```python
from build123d import *

# Parameters (mm, degrees)
ESQUISSE1_R             = 9
BOSS_EXTRU_1_DEPTH      = 23
ESQUISSE2_R             = 9
ESQUISSE2_R_2           = 4.5
ENL_V_MAT_EXTRU_2_DEPTH = 27.286878856
ESQUISSE3_R             = 1.5
ENL_V_MAT_EXTRU_3_DEPTH = 5
ESQUISSE4_R             = 2
ENL_V_MAT_EXTRU_4_DEPTH = 5


with BuildPart() as part:
    # Esquisse1 → Boss.-Extru.1 (new body)
    with BuildSketch(Plane(origin=(0, 0, 0), x_dir=(1, 0, 0), z_dir=(0, 1, 0))):
        with Locations(Location((0, 0, 0), (0, 0, 270))):
            Circle(ESQUISSE1_R)
    extrude(amount=BOSS_EXTRU_1_DEPTH)

    # Esquisse2 → Enlèv. mat.-Extru.2 (cut, through all)
    with BuildSketch(Plane(origin=(0, 0, 0), x_dir=(-1, 0, 0), z_dir=(0, -1, 0))):
        Circle(ESQUISSE2_R)
        with Locations(Location((0, 0, 0), (0, 0, 90))):
            Circle(ESQUISSE2_R_2, mode=Mode.SUBTRACT)
    extrude(amount=-ENL_V_MAT_EXTRU_2_DEPTH, mode=Mode.SUBTRACT)

    # Esquisse3 → Enlèv. mat.-Extru.3 (cut)
    with BuildSketch(Plane(origin=(0, 0, 0), x_dir=(-1, 0, 0), z_dir=(0, -1, 0))):
        with Locations(Location((0, 0, 0), (0, 0, 90))):
            Circle(ESQUISSE3_R)
    extrude(amount=-ENL_V_MAT_EXTRU_3_DEPTH, mode=Mode.SUBTRACT)

    # Esquisse4 → Enlèv. mat.-Extru.4 (cut)
    with BuildSketch(Plane(origin=(0, 23, 0), x_dir=(1, 0, 0), z_dir=(0, 1, 0))):
        with Locations(Location((0, 0, 0), (0, 0, 270))):
            Circle(ESQUISSE4_R)
    extrude(amount=-ENL_V_MAT_EXTRU_4_DEPTH, mode=Mode.SUBTRACT)


solid = part.part
```
The model under review builds one solid part; all positions refer to its coordinate system, in mm. A direction names the side the tool comes from. Round coordinates to 2 decimals unless told otherwise and drop trailing zeros. Write each loop counter-clockwise with the first axis right and the second up, starting at its lowest first coordinate (ties: lowest second). Pieces come first, ordered by that corner, then holes. Notation, with made-up numbers: M 37.25,51 L 52.25,51 A19 cw 52.25,56 Z; hole C 86.25,41 d8. An arc over 180 degrees is marked long. Use CSV: the item, a comma, the result in double quotes. Start each with the question number.
(1) We need section A-A, the plane z = 0. State the section outline as (x, y) points, then the cut area to 3 significant figures.
(2) We need section D-D, the plane y = 15. State the section outline as (x, z) points, then the cut area to 3 significant figures.
(3) For line 1 along X through (y, z) = (1.95, 0); line 2 along X through (y, z) = (20.05, 0); line 3 along Y through (x, z) = (-1.5, 1), list the stretches that pass through material, from the lowest coordinate up.
(4) Tool access review of faces 1 (the face through (-2, 23, 1)), 2 (the face through (0, 5, 0)): name each direction out of +Z, -Z, +X, -X, +Y, -Y from which nothing blocks a thin tool from reaching the whole face with its end or side.
(5) We need section C-C, the plane y = 20.5. State the section outline as (x, z) points, then the cut area to 3 significant figures.
(6) We need section B-B, the plane x = 0. State the section outline as (y, z) points.
(7) Clearance check with flat-ended pins moving along their axes: P1, Ø4, axis at y = 19, z = 3, coming from the -X side; P2, Ø1.2, axis at x = 1, z = 0, coming from the +Y side; P3, Ø1, axis at x = -2.5, y = 3.5, coming from the +Z side. State where each tip first meets the part, or that it passes through.
(8) The part is to be moulded in two halves that separate along Z. For faces 3 (the face through (0, 18, 0)), 4 (the face through (-2, 21, 0)), 5 (the face through (1.352, 11.339, -4.292)), 6 (the face through (-2, 0, 0)), say which applies: +Z half, -Z half, draft (parallel to the pull), parting line (faces both ways), or undercut.
Findings:
1,outline,"M -4.5,0 L -1.5,0 L -1.5,5 L 1.5,5 L 1.5,0 L 4.5,0 L 4.5,23 L 2,23 L 2,18 L -2,18 L -2,23 L -4.5,23 Z"
1,area,"172 mm^2"
2,outline,"C 0,0 d9"
2,area,"63.6 mm^2"
3,line 1,"-4.5 to -1.5, 1.5 to 4.5"
3,line 2,"-4.5 to -2, 2 to 4.5"
3,line 3,"0 to 18"
4,face 1,"+Z, -Z, +X, -X, +Y"
4,face 2,"-Y"
5,outline,"C 0,0 d9; hole C 0,0 d4"
5,area,"51.1 mm^2"
6,outline,"M 0,-4.5 L 23,-4.5 L 23,-2 L 18,-2 L 18,2 L 23,2 L 23,4.5 L 0,4.5 L 0,1.5 L 5,1.5 L 5,-1.5 L 0,-1.5 Z"
7,P1,"x = -4.39"
7,P2,"y = 18"
7,P3,"z = 4.03"
8,face 3,"undercut"
8,face 4,"undercut"
8,face 5,"parting line"
8,face 6,"draft"
